Can you work these out from the model? Positions are in its coordinate system, mm. Face numbers are marked on the shaded views. A direction names the side the tool comes from. Coordinates: 2 decimals unless noted, no trailing zeros. Order: outer loops, then holes, each group sorted by start corner. A loop starts at its lowest first (then second) coordinate and runs counter-clockwise, first axis right, second up. Notation, with made-up numbers: M 79.25,77.5 L 117.25,77.5 A13 cw 117.25,82.5 Z; hole C 62,24 d4. An arc over 180 degrees is marked long. Answer as a JSON object with one key per item and string values.
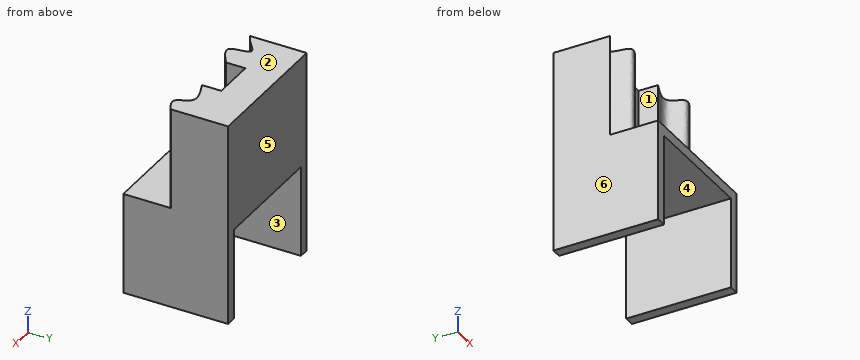
from build123d import *

# Parameters (mm, degrees)
F0_W     = 34.2943547294
F0_H     = 25.8568562567
F1_DEPTH = 25
F2_T     = -2.5
F4_DEPTH = 25


with BuildPart() as f1:
    # F0 (on Top) → F1 (new body)
    with BuildSketch(Plane.XY):
        with Locations((18.5080640949, 12.9284281284)):
            Rectangle(F0_W, F0_H)
    extrude(amount=F1_DEPTH)

    # F2
    f2_openings = [f1.faces().sort_by_distance(p)[0] for p in [
        (18.508064, 25.856856, 12.5),
        (18.508064, 0, 12.5),
        (18.508064, 12.928428, 0),
    ]]
    offset(amount=F2_T, openings=f2_openings)

    # F3 (on face) → F4 (join)
    with BuildSketch(Plane.XY.offset(25)):
        with BuildLine():
            Line((13.2598066702, 17.4573864788), (23.7924046814, 17.4573864788))
            Line((23.7924046814, 17.4573864788), (23.7924046814, 12.689712923))
            add(Edge.make_bspline(
                [(23.7924046814, 12.689712923), (26.3508480961, 13.7881721519), (30.8893318732, 15.7367551698), (31.4069191474, 9.5192493209), (34.1874553016, 10.727986267), (35.6552414596, 11.7030631088)],
                knots=[0, 0, 0, 0, 0.343785498, 0.6098492922, 0.8257809177, 0.8257809177, 0.8257809177, 0.8257809177], degree=3))
            Line((35.6552414596, 11.7030631088), (35.6552414596, 25.8568562567))
            Line((35.6552414596, 25.8568562567), (1.3608867303, 25.8568562567))
            Line((1.3608867303, 25.8568562567), (1.3608867303, 11.8645355105))
            add(Edge.make_bspline(
                [(13.2598066702, 12.689712923), (11.0860272045, 11.1594255192), (6.9288496698, 8.2328745434), (7.8993387733, 18.2466111056), (3.4948427482, 12.7098239865), (1.3608867303, 11.8645355105)],
                knots=[0, 0, 0, 0, 0.2493304721, 0.476824376, 0.7419340081, 0.7419340081, 0.7419340081, 0.7419340081], degree=3))
            Line((13.2598066702, 12.689712923), (13.2598066702, 17.4573864788))
        make_face()
    extrude(amount=F4_DEPTH)


solid = f1.part
Item 1: I want a section at A-A, the plane z = 14. Write out the boundary of the cut face in (x, y), plus the area to 3 significant figures.
Answers follow:
{"outline": "M 1.36,0 L 3.86,0 L 3.86,25.86 L 1.36,25.86 Z; M 33.16,0 L 35.66,0 L 35.66,25.86 L 33.16,25.86 Z", "area": "129 mm^2"}
Item 2: I want a section at C-C, the plane x = 15. Write out the boundary of the cut face in (y, z), plus the area to 3 significant figures.
Answers follow:
{"outline": "M 0,22.5 L 25.86,22.5 L 25.86,50 L 17.46,50 L 17.46,25 L 0,25 Z", "area": "275 mm^2"}
Item 3: If we mould it in two halves opening along X, with no side actions, what happens to the marked faces 4, 5 and 6? For each: pulls with the +X half, pulls with the -X half, needs draft (parallel to the pull), parting line crosses it, or undercut.
Answers follow:
{"face 4": "undercut", "face 5": "needs draft", "face 6": "pulls with the -X half"}
Item 4: I'm going to push flat-ended pins straight in: pin 1 (3 mm diameter, centred on x = 30.5, z = 34, fed in from -Y); pin 2 (12 mm diameter, centred on x = 20, y = 8, fed in from -Z); pin 3 (1 mm diameter, centred on x = 21, y = 16, fed in from +Z). Where does each tip first touch, or does it pass through?
Answers follow:
{"pin 1": "stops at y = 10.76", "pin 2": "stops at z = 22.5", "pin 3": "stops at z = 25"}
Item 5: Please list where these lines run through material, in increasing order: line 1 (X direction, y = 18, z = 4.5); line 2 (X direction, y = 13, z = 40); line 3 (Z direction, x = 17.5, y = 19.5).
Answers follow:
{"line 1": "x = 1.36 to 3.86, 33.16 to 35.66", "line 2": "x = 1.36 to 3.24, 7.41 to 13.26, 23.79 to 24.52, 30.82 to 35.66", "line 3": "z = 22.5 to 50"}
Item 6: I want a section at B-B, the plane y = 16. Write out the boundary of the cut face in (x, z), plus the area to 3 significant figures.
Answers follow:
{"outline": "M 1.36,0 L 3.86,0 L 3.86,22.5 L 33.16,22.5 L 33.16,0 L 35.66,0 L 35.66,50 L 23.79,50 L 23.79,25 L 13.26,25 L 13.26,50 L 1.36,50 Z", "area": "792 mm^2"}
Item 7: Which directions (+Z, -Z, +X, -X, +Y, -Y) give clear straight access to the entire face, cutting with the end or side of a thin tool? Please do the marked faces 1, 2 and 3.
Answers follow:
{"face 1": "+Z, -Y", "face 2": "+Z, +X, -X, +Y, -Y", "face 3": "-Z, +Y, -Y"}
Item 8: I want a section at D-D, the plane y = 3.75. Write out the boundary of the cut face in (x, z), plus the area to 3 significant figures.
Answers follow:
{"outline": "M 1.36,0 L 3.86,0 L 3.86,22.5 L 33.16,22.5 L 33.16,0 L 35.66,0 L 35.66,25 L 1.36,25 Z", "area": "198 mm^2"}
